Geometry: final body of the model. Coordinates: model frame, mm. Give positions to 0.01 mm unless a question says otherwise; leave off trailing zeros. Write each loop counter-clockwise with the first axis right and the second up, starting at its lowest first coordinate (ties: lowest second). Pieces come first, ordered by that corner, then holes. Notation, with made-up numbers: (-36.5, 13) - (-5.5, 13) arc R20 cw to (-5.5, 32) - close; hole circle Ø9 at (29.25, 51.5). An arc over 180 degrees is marked (long way). Return JSON: item names as keys, results as strings.
from build123d import *

# Parameters (mm, degrees)
BOSS_EXTRUDE1_DEPTH   = 1.2
SKETCH8_3_R           = 3
CUT_EXTRUDE1_DEPTH    = 182.287051241
SKETCH16_R            = 1.6
SKETCH16_W            = 18
SKETCH16_H            = 3.2
CUT_EXTRUDE2_DEPTH    = 182.287051241
CUT_EXTRUDE3_DEPTH    = 182.287051241
SKETCH9_W             = 14.1
SKETCH9_H             = 14.1
CUT_EXTRUDE4_DEPTH    = 182.287051241
F_3_0MM_DOWEL_HOLE1_D = 3
FILLET1_R             = 1


with BuildPart() as part:
    # Sketch8 → Boss-Extrude1 (new body)
    with BuildSketch(Plane.XY):
        with BuildLine():
            ThreePointArc((116.356165737, 89.593531525), (107.510169126, 99.635128091), (106.844308874, 113.000828513))
            ThreePointArc((106.844308874, 113.000828513), (98.551785503, 130.943955248), (79.67265081, 125.087333856))
            ThreePointArc((79.67265081, 125.087333856), (66.957923375, 111.551078569), (49.923987164, 104.152462611))
            ThreePointArc((49.923987164, 104.152462611), (38.279791522, 92.371702096), (44.581782069, 77.053134095))
            ThreePointArc((44.581782069, 77.053134095), (58.651333394, 69.17496271), (73.852303576, 63.794594289))
            ThreePointArc((73.852303576, 63.794594289), (73.863549821, 63.839319131), (73.875482243, 63.883865813))
            ThreePointArc((73.875482243, 63.883865813), (76.767270103, 63.085390407), (79.729789892, 62.612657392))
            ThreePointArc((79.729789892, 62.612657392), (79.717062502, 62.538833177), (79.702495752, 62.465349771))
            ThreePointArc((79.702495752, 62.465349771), (95.373691885, 60.7573177), (111.111302129, 61.669121188))
            ThreePointArc((111.111302129, 61.669121188), (123.74416397, 73.75113123), (116.356165737, 89.593531525))
        make_face()
        with BuildLine():
            ThreePointArc((109.375963817, 92.019534234), (109.377797318, 92.017499849), (109.379631064, 92.015465685))
            ThreePointArc((109.379631064, 92.015465685), (109.377986421, 92.015505684), (109.376341775, 92.015545509))
            ThreePointArc((109.376341775, 92.015545509), (109.37615287, 92.017539878), (109.375963817, 92.019534234))
        make_face(mode=Mode.SUBTRACT)
        with BuildLine():
            ThreePointArc((56.72077423, 104.000844147), (56.721683918, 104.00117089), (56.7225936, 104.001497652))
            ThreePointArc((56.7225936, 104.001497652), (56.755397532, 103.992206145), (56.788325126, 103.983362865))
            ThreePointArc((56.788325126, 103.983362865), (56.754559843, 103.992142785), (56.72077423, 104.000844147))
        make_face(mode=Mode.SUBTRACT)
        with BuildLine():
            ThreePointArc((103.532400156, 106.396636288), (103.543227812, 106.407709628), (103.554044399, 106.418793781))
            ThreePointArc((103.554044399, 106.418793781), (103.552293137, 106.396310438), (103.550744757, 106.373812212))
            ThreePointArc((103.550744757, 106.373812212), (103.541575551, 106.385226737), (103.532400156, 106.396636288))
        make_face(mode=Mode.SUBTRACT)
        with BuildLine():
            ThreePointArc((104.104138674, 107.788453533), (104.062244422, 107.735361058), (104.021801646, 107.681154775))
            ThreePointArc((104.021801646, 107.681154775), (104.021865069, 107.684582448), (104.021929019, 107.688010111))
            ThreePointArc((104.021929019, 107.688010111), (104.063142491, 107.7381429), (104.104138674, 107.788453533))
        make_face(mode=Mode.SUBTRACT)
    extrude(amount=BOSS_EXTRUDE1_DEPTH)

    # Sketch8_3 → Cut-Extrude1 (cut, through all)
    with BuildSketch(Plane.XY):
        with Locations((106.04559389, 106.21341333)):
            Circle(SKETCH8_3_R)
        with Locations((76.767270103, 63.085390407)):
            Circle(SKETCH8_3_R)
        with Locations((57.420286528, 106.402169345)):
            Circle(SKETCH8_3_R)
    extrude(amount=CUT_EXTRUDE1_DEPTH, mode=Mode.SUBTRACT)

    # Sketch16 → Cut-Extrude2 (cut, through all)
    with BuildSketch(Plane.XY):
        with Locations((43.996556322, 89.970524089)):
            Circle(SKETCH16_R)
        with Locations((61.996556322, 89.970524089)):
            Circle(SKETCH16_R)
        with Locations((73.496556322, 89.970524089)):
            Circle(SKETCH16_R)
        with Locations((91.496556322, 89.970524089)):
            Circle(SKETCH16_R)
        with Locations((100.001946024, 77.020067852)):
            Circle(SKETCH16_R)
        with Locations((118.001946024, 77.020067852)):
            Circle(SKETCH16_R)
        with Locations((83.45540719, 117.738694526)):
            Circle(SKETCH16_R)
        with Locations((101.45540719, 117.738694526)):
            Circle(SKETCH16_R)
        with Locations((52.996556322, 89.970524089)):
            Rectangle(SKETCH16_W, SKETCH16_H)
        with Locations((82.496556322, 89.970524089)):
            Rectangle(SKETCH16_W, SKETCH16_H)
        with Locations((109.001946024, 77.020067852)):
            Rectangle(SKETCH16_W, SKETCH16_H)
        with Locations((92.45540719, 117.738694526)):
            Rectangle(SKETCH16_W, SKETCH16_H)
    extrude(amount=CUT_EXTRUDE2_DEPTH, mode=Mode.SUBTRACT)

    # Sketch14 → Cut-Extrude3 (cut, through all)
    with BuildSketch(Plane.XY):
        with BuildLine():
            Line((45.946556322, 95.106310527), (47.360769884, 96.520524089))
            ThreePointArc((47.360769884, 96.520524089), (45.946556322, 96.520524089), (45.946556322, 95.106310527))
        make_face()
        with BuildLine():
            Line((45.946556322, 83.834737652), (47.360769884, 82.420524089))
            ThreePointArc((47.360769884, 82.420524089), (45.946556322, 82.420524089), (45.946556322, 83.834737652))
        make_face()
        with BuildLine():
            Line((58.63234276, 82.420524089), (60.046556322, 83.834737652))
            ThreePointArc((60.046556322, 83.834737652), (60.046556322, 82.420524089), (58.63234276, 82.420524089))
        make_face()
        with BuildLine():
            Line((58.63234276, 96.520524089), (60.046556322, 95.106310527))
            ThreePointArc((60.046556322, 95.106310527), (60.046556322, 96.520524089), (58.63234276, 96.520524089))
        make_face()
        with BuildLine():
            Line((85.40540719, 111.602908088), (86.819620752, 110.188694526))
            ThreePointArc((86.819620752, 110.188694526), (85.40540719, 110.188694526), (85.40540719, 111.602908088))
        make_face()
        with BuildLine():
            Line((98.091193628, 110.188694526), (99.50540719, 111.602908088))
            ThreePointArc((99.50540719, 111.602908088), (99.50540719, 110.188694526), (98.091193628, 110.188694526))
        make_face()
        with BuildLine():
            Line((98.091193628, 124.288694526), (99.50540719, 122.874480963))
            ThreePointArc((99.50540719, 122.874480963), (99.50540719, 124.288694526), (98.091193628, 124.288694526))
        make_face()
        with BuildLine():
            Line((85.40540719, 122.874480963), (86.819620752, 124.288694526))
            ThreePointArc((86.819620752, 124.288694526), (85.40540719, 124.288694526), (85.40540719, 122.874480963))
        make_face()
        with BuildLine():
            Line((101.951946024, 82.155854289), (103.366159586, 83.570067852))
            ThreePointArc((103.366159586, 83.570067852), (101.951946024, 83.570067852), (101.951946024, 82.155854289))
        make_face()
        with BuildLine():
            Line((101.951946024, 70.884281414), (103.366159586, 69.470067852))
            ThreePointArc((103.366159586, 69.470067852), (101.951946024, 69.470067852), (101.951946024, 70.884281414))
        make_face()
        with BuildLine():
            Line((114.637732461, 69.470067852), (116.051946024, 70.884281414))
            ThreePointArc((116.051946024, 70.884281414), (116.051946024, 69.470067852), (114.637732461, 69.470067852))
        make_face()
        with BuildLine():
            Line((116.051946024, 82.155854289), (114.637732461, 83.570067852))
            ThreePointArc((114.637732461, 83.570067852), (116.051946024, 83.570067852), (116.051946024, 82.155854289))
        make_face()
        with BuildLine():
            Line((76.860769884, 96.520524089), (75.446556322, 95.106310527))
            ThreePointArc((75.446556322, 95.106310527), (75.446556322, 96.520524089), (76.860769884, 96.520524089))
        make_face()
        with BuildLine():
            Line((88.13234276, 96.520524089), (89.546556322, 95.106310527))
            ThreePointArc((89.546556322, 95.106310527), (89.546556322, 96.520524089), (88.13234276, 96.520524089))
        make_face()
        with BuildLine():
            Line((89.546556322, 83.834737652), (88.13234276, 82.420524089))
            ThreePointArc((88.13234276, 82.420524089), (89.546556322, 82.420524089), (89.546556322, 83.834737652))
        make_face()
        with BuildLine():
            Line((75.446556322, 83.834737652), (76.860769884, 82.420524089))
            ThreePointArc((76.860769884, 82.420524089), (75.446556322, 82.420524089), (75.446556322, 83.834737652))
        make_face()
    extrude(amount=CUT_EXTRUDE3_DEPTH, mode=Mode.SUBTRACT)

    # Sketch9 → Cut-Extrude4 (cut, through all)
    with BuildSketch(Plane.XY):
        with Locations((52.996556322, 89.470524089)):
            Rectangle(SKETCH9_W, SKETCH9_H)
        with Locations((82.496556322, 89.470524089)):
            Rectangle(SKETCH9_W, SKETCH9_H)
        with Locations((109.001946024, 76.520067852)):
            Rectangle(SKETCH9_W, SKETCH9_H)
        with Locations((92.45540719, 117.238694526)):
            Rectangle(SKETCH9_W, SKETCH9_H)
    extrude(amount=CUT_EXTRUDE4_DEPTH, mode=Mode.SUBTRACT)

    # 3.0mm Dowel Hole1 (through all)
    with Locations(Plane.XY.offset(1.2)):
        with Locations((70.435309654, 103.157249982)):
            Hole(F_3_0MM_DOWEL_HOLE1_D / 2)

    # Fillet1
    fillet1_edges = [part.edges().sort_by_distance(p)[0] for p in [
        (106.42311517, 103.237261841, 0.6),
        (106.111211206, 109.212695638, 0.6),
        (54.596217873, 105.389926178, 0.6),
        (60.17229201, 107.596516793, 0.6),
        (73.852303576, 63.794594289, 0.6),
        (79.702495752, 62.465349771, 0.6),
    ]]
    fillet(fillet1_edges, radius=FILLET1_R)


solid = part.part
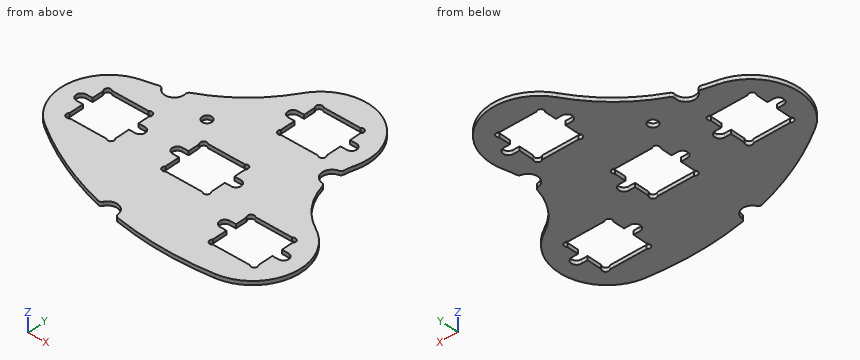
Q1. Section query D-D, the plane y = 128.5. Return the cut outline in (x, z), plus the area to 3 significant figures.
Answer key:
{"outline": "(82.55, 0) - (102.36, 0) - (102.36, 1.2) - (82.55, 1.2) - close", "area": "23.8 mm^2"}
Q2. Section query B-B, the plane y = 93.5. Return the cut outline in (x, z).
Answer key:
{"outline": "(38.55, 0) - (45.95, 0) - (45.95, 1.2) - (38.55, 1.2) - close; (60.05, 0) - (75.45, 0) - (75.45, 1.2) - (60.05, 1.2) - close; (89.55, 0) - (111.41, 0) - (111.41, 1.2) - (89.55, 1.2) - close"}
Q3. Section query A-A, the plane y = 80.5. Return the cut outline in (x, z).
Answer key:
{"outline": "(40.97, 0) - (101.95, 0) - (101.95, 1.2) - (40.97, 1.2) - close; (116.05, 0) - (123.46, 0) - (123.46, 1.2) - (116.05, 1.2) - close"}
Q4. Material intervals for probe 1 along X at (y, z) = (85.5, 0.2); probe 2 along X at (y, z) = (93, 0.3); probe 3 along Y at (x, z) = (99, 0.8), sorted ascending. Write a range as [from, to].
Answer key:
{"probe 1": "x = [38.53, 45.95], [60.05, 75.45], [89.55, 121.02]", "probe 2": "x = [38.42, 45.95], [60.05, 75.45], [89.55, 111.89]", "probe 3": "y = [60.73, 75.77], [78.27, 109.92], [124.56, 130.74]"}
Q5. Pin query (flat end, axial travel): P1, Ø0.6, axis at x = 61, z = 0.5, coming from the +Y side. Return the tip coordinate at first contact, or that it passes through.
Answer key:
{"P1": "stops at y = 108.15"}
